Model file for the job. Use its own axes, mm. A direction names the side the tool comes from. Round coordinates to 2 decimals unless told otherwise and drop trailing zeros. Order: outer loops, then holes, each group sorted by start corner. A loop starts at its lowest first (then second) coordinate and runs counter-clockwise, first axis right, second up. Notation, with made-up numbers: M 52.5,23.5 L 73.5,23.5 A34 cw 73.5,59.5 Z; hole C 23.5,84.5 d1. An arc over 180 degrees is marked long. Return JSON: item names as keys, results as strings. Group by question number.
Item 1: Probe line 1 along X through (y, z) = (1.3, 0); line 2 along Z through (x, y) = (10, 2.4); line 3 along Z through (x, y) = (-6.5, 2.15). List the from-to ranges inside material, lowest first.
Item 2: Pull direction Z, two halves, no side cores. Call faces 1 (the face through (26.5, 0, -35.6)), 2 (the face through (-11.99, 1.48, -87.85)), 3 (the face through (19.637, 1.479, -58.309)), 4 (the face through (36.542, 1.479, -44.139)): pulls with the +Z half, pulls with the -Z half, needs draft (parallel to the pull), parting line crosses it, or undercut.
Item 3: Which spindle directions (+Z, -Z, +X, -X, +Y, -Y) get a long thin tool onto all of the face, cutting with end or side? Do faces 5 (the face through (5, 1, -72)), 6 (the face through (22.488, 1.479, -22.788)). Say none if no direction does.
Item 4: Pin check, flat tip, straight feed: pin 1 Ø1.8 at (x, z) = (29.37, -52.81) entering from -Y. Stop position of the tip, or through.
Item 5: Slice it at A-A on z = 0. Write the cut outline in (x, y).
Item 6: Slice it at B-B on y = 1.4. Give the number of separate pieces and of enclosed holes in the cut face, then the cut area to 3 significant figures.
from build123d import *

# Parameters (mm, degrees)
SKETCH_1_R          = 1.5
EXTRUDE_1_DEPTH     = 3
SKETCH_2_R          = 1.5
CUT_EXTRUDE_1_DEPTH = 35
SKETCH_3_R          = 1.5
CUT_EXTRUDE_2_DEPTH = 10


with BuildPart() as part:
    # 草图1 → 凸台-拉伸1 (new body)
    with BuildSketch(Plane(origin=(0, 0, 0), x_dir=(1, 0, 0), z_dir=(0, 1, 0))):
        with BuildLine():
            Line((-11.919787954, 77.793366188), (-10.248955421, 74.860550413))
            Line((-10.248955421, 74.860550413), (-8.665067312, 77.567824645))
            ThreePointArc((-8.665067312, 77.567824645), (-8.552157803, 77.555194327), (-8.439284624, 77.542243357))
            Line((-8.439284624, 77.542243357), (-7.03042185, 74.474965181))
            Line((-7.03042185, 74.474965181), (-5.216606417, 77.033892473))
            ThreePointArc((-5.216606417, 77.033892473), (-5.105227368, 77.011469504), (-4.993912457, 76.988730272))
            Line((-4.993912457, 76.988730272), (-3.857741739, 73.810333533))
            Line((-3.857741739, 73.810333533), (-1.827803212, 76.201438903))
            ThreePointArc((-1.827803212, 76.201438903), (-1.718802284, 76.169393937), (-1.609892815, 76.1370395))
            Line((-1.609892815, 76.1370395), (-0.755061098, 72.871713718))
            Line((-0.755061098, 72.871713718), (1.475551464, 75.07679941))
            ThreePointArc((1.475551464, 75.07679941), (1.581344708, 75.035376328), (1.687019869, 74.993652924))
            Line((1.687019869, 74.993652924), (2.254006799, 71.666249199))
            Line((2.254006799, 71.666249199), (4.668317088, 73.66853318))
            ThreePointArc((4.668317088, 73.66853318), (4.770097497, 73.618047236), (4.871734098, 73.567272405))
            Line((4.871734098, 73.567272405), (5.146561129, 70.203114289))
            Line((5.146561129, 70.203114289), (7.726194786, 71.987357968))
            ThreePointArc((7.726194786, 71.987357968), (7.82318775, 71.928193392), (7.920012274, 71.868753561))
            Line((7.920012274, 71.868753561), (7.900587806, 68.493444328))
            Line((7.900587806, 68.493444328), (10.625912261, 70.046068534))
            ThreePointArc((10.625912261, 70.046068534), (10.717379605, 69.978675602), (10.808655161, 69.911023145))
            Line((10.808655161, 69.911023145), (10.495127025, 66.550250936))
            Line((10.495127025, 66.550250936), (13.345400914, 67.859439261))
            ThreePointArc((13.345400914, 67.859439261), (13.430646516, 67.784330876), (13.51567844, 67.708980668))
            Line((13.51567844, 67.708980668), (12.910432776, 64.38832299))
            Line((12.910432776, 64.38832299), (15.863963793, 65.44411172))
            ThreePointArc((15.863963793, 65.44411172), (15.942338882, 65.361859501), (16.020480031, 65.279385002))
            Line((16.020480031, 65.279385002), (15.128123123, 62.024114065))
            Line((15.128123123, 62.024114065), (18.162433114, 62.818468011))
            ThreePointArc((18.162433114, 62.818468011), (18.233341209, 62.729697948), (18.303996881, 62.640726839))
            Line((18.303996881, 62.640726839), (17.131320104, 59.47561722))
            Line((17.131320104, 59.47561722), (20.223316137, 60.002490868))
            ThreePointArc((20.223316137, 60.002490868), (20.286217585, 59.907878554), (20.348850048, 59.81308796))
            Line((20.348850048, 59.81308796), (18.90477818, 56.762228053))
            Line((18.90477818, 56.762228053), (22.030928299, 57.017611578))
            ThreePointArc((22.030928299, 57.017611578), (22.085344382, 56.917877069), (22.139476964, 56.817988403))
            Line((22.139476964, 56.817988403), (20.435000265, 53.904597096))
            Line((20.435000265, 53.904597096), (23.57151258, 53.886546873))
            ThreePointArc((23.57151258, 53.886546873), (23.617029157, 53.782449211), (23.662249878, 53.678222686))
            Line((23.662249878, 53.678222686), (21.710340444, 50.924472645))
            Line((21.710340444, 50.924472645), (24.833344202, 50.633126049))
            ThreePointArc((24.833344202, 50.633126049), (24.869614866, 50.525457478), (24.905579569, 50.417686321))
            Line((24.905579569, 50.417686321), (22.721092609, 47.844535247))
            Line((22.721092609, 47.844535247), (25.806819865, 47.2821096))
            ThreePointArc((25.806819865, 47.2821096), (25.833568575, 47.171689544), (25.860003545, 47.061193959))
            Line((25.860003545, 47.061193959), (23.459564325, 44.688225085))
            Line((23.459564325, 44.688225085), (26.484530833, 43.859000786))
            ThreePointArc((26.484530833, 43.859000786), (26.501554013, 43.746669609), (26.518258066, 43.634290532))
            Line((26.518258066, 43.634290532), (23.920135376, 41.479563585))
            Line((23.920135376, 41.479563585), (26.861319314, 40.389851532))
            ThreePointArc((26.861319314, 40.389851532), (26.868487408, 40.276464141), (26.875333415, 40.163056847))
            Line((26.875333415, 40.163056847), (24.09930054, 38.242970598))
            Line((24.09930054, 38.242970598), (26.934317721, 36.901064158))
            ThreePointArc((26.934317721, 36.901064158), (26.931576177, 36.7874835), (26.928512036, 36.673911086))
            Line((26.928512036, 36.673911086), (23.99569626, 35.003078552))
            Line((23.99569626, 35.003078552), (26.702970493, 33.419190443))
            ThreePointArc((26.702970493, 33.419190443), (26.690340174, 33.306280935), (26.677389205, 33.193407756))
            Line((26.677389205, 33.193407756), (23.610111028, 31.784544982))
            Line((23.610111028, 31.784544982), (26.16903832, 29.970729549))
            ThreePointArc((26.16903832, 29.970729549), (26.146615352, 29.8593505), (26.123876119, 29.748035589))
            Line((26.123876119, 29.748035589), (22.945479381, 28.611864871))
            Line((22.945479381, 28.611864871), (25.336584751, 26.581926344))
            ThreePointArc((25.336584751, 26.581926344), (25.304539784, 26.472925416), (25.272185348, 26.364015947))
            Line((25.272185348, 26.364015947), (22.006859566, 25.50918423))
            Line((22.006859566, 25.50918423), (24.211945258, 23.278571668))
            ThreePointArc((24.211945258, 23.278571668), (24.170522175, 23.172778424), (24.128798771, 23.067103263))
            Line((24.128798771, 23.067103263), (20.801395047, 22.500116333))
            Line((20.801395047, 22.500116333), (22.803679027, 20.085806044))
            ThreePointArc((22.803679027, 20.085806044), (22.753193083, 19.984025635), (22.702418252, 19.882389034))
            Line((22.702418252, 19.882389034), (19.338260136, 19.607562003))
            Line((19.338260136, 19.607562003), (21.122503815, 17.027928346))
            ThreePointArc((21.122503815, 17.027928346), (21.063339239, 16.930935382), (21.003899408, 16.834110857))
            Line((21.003899408, 16.834110857), (17.628590175, 16.853535326))
            Line((17.628590175, 16.853535326), (19.181214381, 14.12821087))
            ThreePointArc((19.181214381, 14.12821087), (19.11382145, 14.036743527), (19.046168992, 13.945467971))
            Line((19.046168992, 13.945467971), (15.685396784, 14.258996107))
            Line((15.685396784, 14.258996107), (16.994585109, 11.408722218))
            ThreePointArc((16.994585109, 11.408722218), (16.919476724, 11.323476616), (16.844126515, 11.238444692))
            Line((16.844126515, 11.238444692), (13.523468837, 11.843690356))
            Line((13.523468837, 11.843690356), (14.579257567, 8.890159339))
            ThreePointArc((14.579257567, 8.890159339), (11.875157779, 6.528999379), (8.970254591, 4.419788747))
            ThreePointArc((8.970254591, 4.419788747), (-9.248107271, 3.804275476), (3.263841378, -9.452372161))
            ThreePointArc((3.263841378, -9.452372161), (36.41039757, 45.099089654), (-11.063458372, 87.769795947))
            Line((-11.063458372, 87.769795947), (-12.946912918, 87.931462784))
            Line((-12.946912918, 87.931462784), (-13.8032425, 77.955033025))
            Line((-13.8032425, 77.955033025), (-11.919787954, 77.793366188))
        make_face()
        with Locations(Location((0, 0, 0), (0, 0, 270))):
            Circle(SKETCH_1_R, mode=Mode.SUBTRACT)
    extrude(amount=EXTRUDE_1_DEPTH)

    # 草图2 → 切除-拉伸1 (cut)
    with BuildSketch(Plane(origin=(0, 3, 0), x_dir=(1, 0, 0), z_dir=(0, 1, 0))):
        with Locations(Location((-3.307239505, 7.284378275, 0), (0, 0, 270))):
            Circle(SKETCH_2_R)
        with Locations(Location((3.307239505, -7.284378275, 0), (0, 0, 270))):
            Circle(SKETCH_2_R)
    extrude(amount=-CUT_EXTRUDE_1_DEPTH, mode=Mode.SUBTRACT)

    # 草图3 → 切除-拉伸2 (cut)
    with BuildSketch(Plane(origin=(0, 3, 0), x_dir=(1, 0, 0), z_dir=(0, 1, 0))):
        with Locations(Location((30.819456427, 27.809488642, 0), (0, 0, 270))):
            Circle(SKETCH_3_R)
        with Locations(Location((29.371041361, 52.809488642, 0), (0, 0, 270))):
            Circle(SKETCH_3_R)
    extrude(amount=-CUT_EXTRUDE_2_DEPTH, mode=Mode.SUBTRACT)


solid = part.part
Output values:
{
 "1": {"line 1": "-10 to -1.5, 1.5 to 19.66", "line 2": "-82.18 to -69.69, -5.12 to 6.56", "line 3": "-87.38 to -75.22, -7.6 to 7.6"},
 "2": {"face 1": "needs draft", "face 2": "pulls with the -Z half", "face 3": "undercut", "face 4": "parting line crosses it"},
 "3": {"face 5": "+Y, -Y", "face 6": "-X, +Y, -Y"},
 "4": {"pin 1": "through"},
 "5": {"outline": "M -10,0 L -1.5,0 L -1.5,3 L -10,3 Z; M 1.5,0 L 19.66,0 L 19.66,3 L 1.5,3 Z"},
 "6": {"separate pieces": "1", "enclosed holes": "5", "area": "1,590 mm²"}
}
